Part model, mm, in its own coordinate system. Round coordinates to 2 decimals unless told otherwise and drop trailing zeros. Write each loop counter-clockwise with the first axis right and the second up, starting at its lowest first coordinate (ties: lowest second). Pieces come first, ordered by that corner, then holes. Notation, with made-up numbers: M 33.5,35 L 88.5,35 A11 ccw 88.5,50 Z; hole C 60,25 d6. An arc over 180 degrees is marked long. Use a Markdown table: item, result. Add a question column.
1) Slice it at D-D on y = -9.25. Write the cut outline in (x, z).
2) Two-plate mould, pull along Z, no slides. Class faces 1 (the face through (-7, -4, -5)), 2 (the face through (8, -1, 4)), 3 (the face through (13, -2.4, 5)), 4 (the face through (13.22, -9.1, -0.14)): released by +Z, released by -Z, zero draft, split by the parting line, or undercut.
3) Drop flat-ended pins along their axis: P1, Ø4, axis at x = -3, z = 8, coming from the -Y side; P2, Ø3, axis at x = -4.5, z = 14, coming from the -Y side; P3, Ø6.5, axis at x = 11.5, z = 4, coming from the +Y side. Give the stop position or say it passes through.
4) Wall check: probe 1 along Z at (x, y) = (11.5, -1.5); probe 2 along Z at (x, y) = (11.5, -6.75); probe 3 along X at (y, z) = (-7, 4). Give the ranges that are in metal, low to high.
```python
from build123d import *

# Parameters (mm, degrees)
SKETCH1_W                                = 57
SKETCH1_H                                = 40
BOSS_EXTRUDE1_DEPTH                      = 4
SKETCH2_W                                = 31
SKETCH2_H                                = 21
BOSS_EXTRUDE2_DEPTH                      = 6
CBORE_FOR_M3_PAN_HEAD_SCREW1_D           = 3.2
CBORE_FOR_M3_PAN_HEAD_SCREW1_CBORE_D     = 7
CBORE_FOR_M3_PAN_HEAD_SCREW1_CBORE_DEPTH = 2.4
FILLET1_R                                = 3


with BuildPart() as part:
    # Sketch1 → Boss-Extrude1 (new body)
    with BuildSketch(Plane(origin=(0, 0, 0), x_dir=(1, 0, 0), z_dir=(0, 1, 0))):
        Rectangle(SKETCH1_W, SKETCH1_H)
    extrude(amount=-BOSS_EXTRUDE1_DEPTH)

    # Sketch2 → Boss-Extrude2 (add)
    with BuildSketch(Plane.XZ.offset(4)):
        with Locations((13, 9.5)):
            Rectangle(SKETCH2_W, SKETCH2_H)
    extrude(amount=BOSS_EXTRUDE2_DEPTH)

    # CBORE for M3 Pan Head Screw1 (through all)
    with Locations(Plane(origin=(0, 0, 0), x_dir=(1, 0, 0), z_dir=(0, 1, 0))):
        with Locations((11.5, -4)):
            CounterBoreHole(CBORE_FOR_M3_PAN_HEAD_SCREW1_D / 2, CBORE_FOR_M3_PAN_HEAD_SCREW1_CBORE_D / 2, CBORE_FOR_M3_PAN_HEAD_SCREW1_CBORE_DEPTH)

    # Fillet1
    fillet1_edges = [part.edges().sort_by_distance(p)[0] for p in [
        (13, -10, -1),
        (-2.5, -10, 9.5),
        (13, -4, -1),
        (-2.5, -4, 9.5),
        (-28.5, -2, 20),
        (-28.5, -2, -20),
    ]]
    fillet(fillet1_edges, radius=FILLET1_R - 0.0001)  # a hair under: the kernel refuses the full size


solid = part.part
```
Entries:
| question | item | result |
|---|---|---|
| 1 | outline | M -1.48,0.02 L 28.5,0.02 L 28.5,20 L -1.48,20 Z; hole C 11.5,4 d3.2 |
| 2 | face 1 | zero draft |
| 2 | face 2 | undercut |
| 2 | face 3 | undercut |
| 2 | face 4 | released by -Z |
| 3 | P1 | stops at y = -9.6 |
| 3 | P2 | stops at y = -5.34 |
| 3 | P3 | stops at y = -2.4 |
| 4 | probe 1 | z = -20 to 0.5, 7.5 to 20 |
| 4 | probe 2 | z = -1.01 to 2.4, 5.6 to 20 |
| 4 | probe 3 | x = -2.5 to 9.9, 13.1 to 28.5 |
